```python
from build123d import *

# Parameters (mm, degrees)
SKETCH1_R           = 11.5
BOSS_EXTRUDE1_DEPTH = 2
CHAMFER1_SIZE       = 1.5
SKETCH3_R           = 9
CUT_EXTRUDE1_DEPTH  = 2
CHAMFER2_SIZE       = 1
FILLET1_R           = 0.3
FILLET2_R           = 0.1


with BuildPart() as part:
    # Sketch1 → Boss-Extrude1 (new body)
    with BuildSketch(Plane.XY):
        Circle(SKETCH1_R)
    extrude(amount=BOSS_EXTRUDE1_DEPTH)

    # Chamfer1
    chamfer1_edges = [part.edges().sort_by_distance(p)[0] for p in [
        (-11.5, 0, 0),
    ]]
    chamfer(chamfer1_edges, length=CHAMFER1_SIZE)

    # Sketch3 → Cut-Extrude1 (cut)
    with BuildSketch(Plane.XY.offset(2)):
        Circle(SKETCH3_R)
    extrude(amount=-CUT_EXTRUDE1_DEPTH, mode=Mode.SUBTRACT)

    # Chamfer2
    chamfer2_edges = [part.edges().sort_by_distance(p)[0] for p in [
        (-9, 0, 2),
    ]]
    chamfer(chamfer2_edges, length=CHAMFER2_SIZE)

    # Fillet1
    fillet1_edges = [part.edges().sort_by_distance(p)[0] for p in [
        (-9, 0, 1),
        (-10, 0, 2),
    ]]
    fillet(fillet1_edges, radius=FILLET1_R)

    # Fillet2
    fillet2_edges = [part.edges().sort_by_distance(p)[0] for p in [
        (-11.5, 0, 2),
    ]]
    fillet(fillet2_edges, radius=FILLET2_R)


solid = part.part
```
For this review, take the finished solid that the model builds, in its own axes (mm). Round coordinates to 2 decimals unless told otherwise and drop trailing zeros.
Q1. To check wall thickness, follow line 1 along Y through (x, z) = (-3.5, 1.65); line 2 along X through (y, z) = (-7.75, 0.8); line 3 along Y through (x, z) = (0, 0.4). State the ranges of each line that lie inside material, in increasing order.
Result sheet:
line 1: y = -10.95 to -8.99, 8.99 to 10.95
line 2: x = -7.52 to -4.58, 4.58 to 7.52
line 3: y = -10.4 to -9, 9 to 10.4
Q2. Mouldability with a two-part tool opening along Y and no side actions: class faces 1 (the face through (-1.5, 11.4, 1.7)), 2 (the face through (8.584, 2.703, 0.444)), 3 (the face through (-9, 2, 0)) as +Y half, -Y half, draft (parallel to the pull), parting line (faces both ways), or undercut.
Result sheet:
face 1: parting line
face 2: undercut
face 3: draft
Q3. Insertion check: pin 1 Ø1 at (x, z) = (8, 0.5) entering from -Y. The pin has a flat end and moves straight along its axis. Give the tip position at first contact, or say it passes through.
Result sheet:
pin 1: stops at y = -7.72
